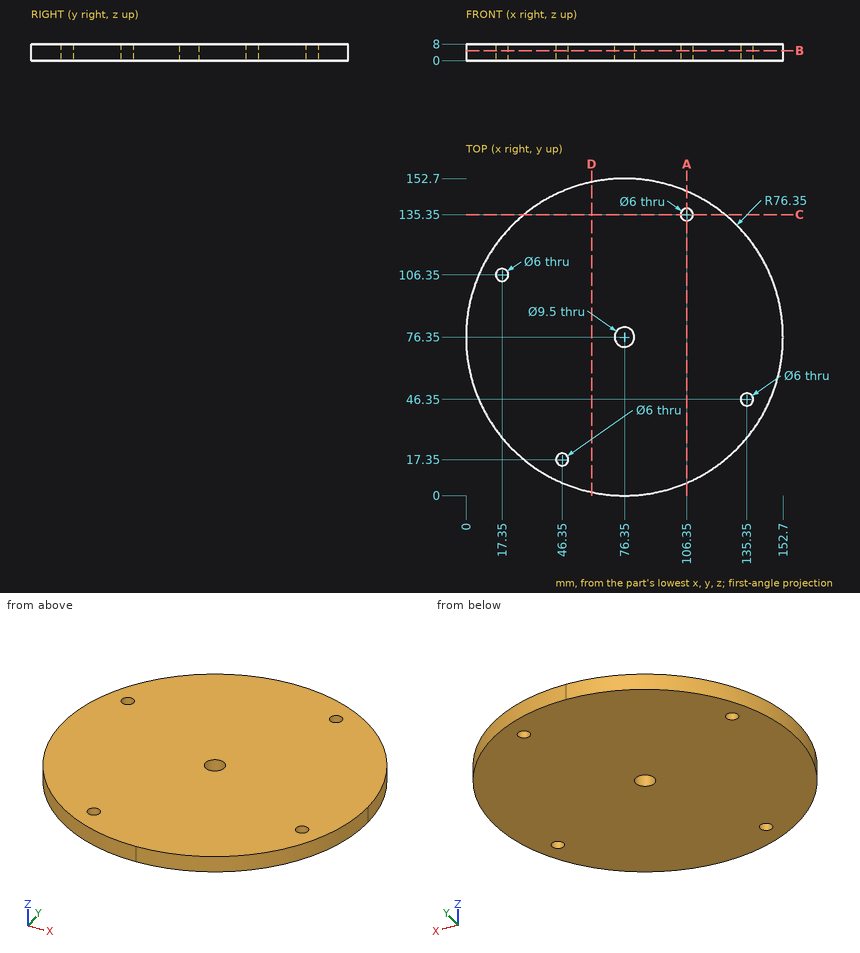
Can you work these out from the drawing? Everything is in mm from the part's minimum corner. Give positions to 0.01 mm unless a question says otherwise; leave off trailing zeros. Loops run counter-clockwise (first coordinate to the right, second up) from the corner with the lowest first, then second, coordinate; pieces in that order, holes last. Notation, with made-up numbers: (32.5, -10) - (90.5, -10) arc R9 ccw to (90.5, -5) - close; hole circle Ø2 at (41.25, -39). An arc over 180 degrees is marked (long way). Answer as a JSON object with one key per item and string values.
Q1. Imagine slicing it at D-D on x = 60.5. Write out the boundary of the cut face in (y, z), plus the area to 3 significant figures.
Geometry says:
{"outline": "(1.66, 0) - (151.04, 0) - (151.04, 8) - (1.66, 8) - close", "area": "1,190 mm²"}
Q2. Imagine slicing it at A-A on x = 106.35. Write out the boundary of the cut face in (y, z).
Geometry says:
{"outline": "(6.14, 0) - (132.35, 0) - (132.35, 8) - (6.14, 8) - close; (138.35, 0) - (146.56, 0) - (146.56, 8) - (138.35, 8) - close"}
Q3. Imagine slicing it at B-B on z = 4.75. Write out the boundary of the cut face in (x, y).
Geometry says:
{"outline": "circle Ø152.7 at (76.35, 76.35); hole circle Ø6 at (17.35, 106.35); hole circle Ø6 at (46.35, 17.35); hole circle Ø9.5 at (76.35, 76.35); hole circle Ø6 at (106.35, 135.35); hole circle Ø6 at (135.35, 46.35)"}
Q4. Will these pins go through, and if not, where does the flat tip stop? P1, Ø3, axis at y = 46, z = 4.5, coming from the -X side; P2, Ø1.5, axis at y = 109.5, z = 6, coming from the +X side; P3, Ø3, axis at y = 67.5, z = 6.5, coming from the -X side.
Geometry says:
{"P1": "x = 5.66", "P2": "x = 145.48", "P3": "x = 0.35"}
Q5. Imagine slicing it at C-C on y = 135.35. Write out the boundary of the cut face in (x, z).
Geometry says:
{"outline": "(27.89, 0) - (103.35, 0) - (103.35, 8) - (27.89, 8) - close; (109.35, 0) - (124.81, 0) - (124.81, 8) - (109.35, 8) - close"}
Q6. If I drill on L1, parallel to Y at x = 76.35, z = 6; L2, parallel to Y at x = 79.5, z = 6.5 (3 decimals); L3, parallel to X at y = 133.5, z = 1.5, over which ranges is the centre line in solid material (lowest first)?
Geometry says:
{"L1": "0 to 71.6, 81.1 to 152.7", "L2": "0.065 to 72.795, 79.905 to 152.635", "L3": "25.72 to 103.99, 108.71 to 126.98"}
